Geometry check sheet. Reference: drawing and pictorial views, mm from the part's lowest x, y, z. Give positions to 0.01 mm unless a question says otherwise; leave off trailing zeros. Loops run counter-clockwise (first coordinate to the right, second up) from the corner with the lowest first, then second, coordinate; pieces in that order, holes last. Notation, with made-up numbers: (14.25, -19) -> (59.25, -19) arc R32 cw to (59.25, 9) -> close; hole circle Ø7 at (-39, 37.25). An arc over 180 degrees is marked (long way). Write item = value, one per line. Start each with the question number.
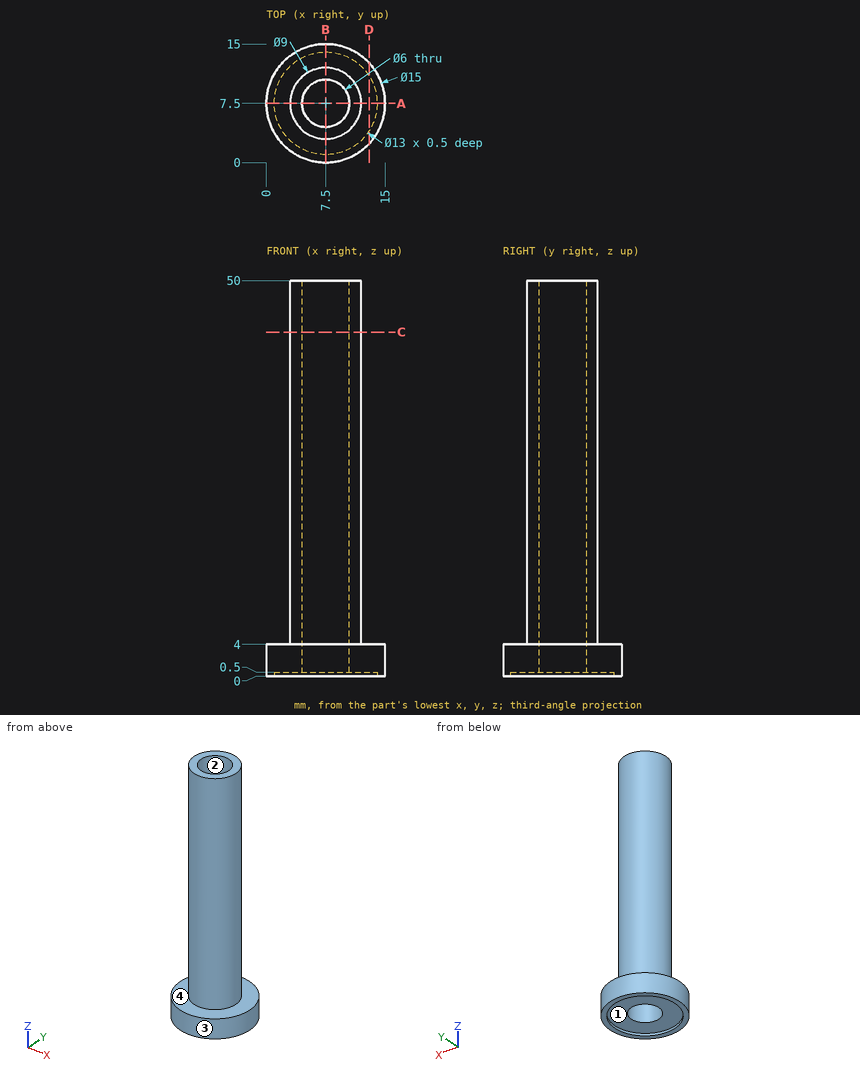
1) Section check D-D (x = 13). Enter the section's corners in (y, z), plus the area to 3 significant figures.
2) Thickness scan on line 1 (X direction, y = 7.5, z = 22.5); line 2 (X direction, y = 7.5, z = 0.25); line 3 (Y direction, x = 8.25, z = 35). Record the ranges inside material, lowest first.
3) Draft check along Y on the marked faces 1, 2, 3 and 4. Enter one of: released by +Y, released by -Y, zero draft, split by the parting line, or undercut.
4) Section check A-A (y = 7.5). Enter the section's corners in (x, z).
5) Depth check by flat-ended pin: pin 1 Ø4.5 at (x, y) = (7.5, 8) entering from +Z; pin 2 Ø2 at (x, z) = (10, 8) entering from -Y; pin 3 Ø4 at (x, z) = (9.5, 41.5) entering from +Y; pin 4 Ø1.5 at (x, y) = (9.5, 11) entering from -Z. Enter the tip coordinate at first touch or a pass-through.
6) Section check C-C (z = 43.5). Enter the section's corners in (x, y), plus the area to 3 significant figures.
Check result:
q1.outline = (2.4, 0) -> (4.04, 0) -> (4.04, 0.5) -> (10.96, 0.5) -> (10.96, 0) -> (12.6, 0) -> (12.6, 4) -> (2.4, 4) -> close
q1.area = 37.3 mm2
q2.line_1 = 3 to 4.5, 10.5 to 12
q2.line_2 = 0 to 1, 14 to 15
q2.line_3 = 3.06 to 4.6, 10.4 to 11.94
q3.face_1 = undercut
q3.face_2 = undercut
q3.face_3 = split by the parting line
q3.face_4 = zero draft
q4.outline = (0, 0) -> (1, 0) -> (1, 0.5) -> (4.5, 0.5) -> (4.5, 50) -> (3, 50) -> (3, 4) -> (0, 4) -> close; (10.5, 0.5) -> (14, 0.5) -> (14, 0) -> (15, 0) -> (15, 4) -> (12, 4) -> (12, 50) -> (10.5, 50) -> close
q5.pin_1 = through
q5.pin_2 = 3.26
q5.pin_3 = 12
q5.pin_4 = 0.5
q6.outline = circle Ø9 at (7.5, 7.5); hole circle Ø6 at (7.5, 7.5)
q6.area = 35.3 mm2
